```python
from build123d import *

# Parameters (mm, degrees)
BOSS_EXTRUDE1_DEPTH    = 24
F_6_0MM_DOWEL_HOLE1_D  = 6
SKETCH4_W              = 32.5
SKETCH4_H              = 30.5
CUT_EXTRUDE1_DEPTH     = 2
FILLET1_R              = 2
CUT_EXTRUDE2_DEPTH     = 57.482298112
FILLET2_R              = 4
SKETCH6_W              = 22.5
SKETCH6_H              = 20.5
CUT_EXTRUDE5_DEPTH     = 39.861935104
FILLET3_R              = 4
CUT_EXTRUDE6_DEPTH     = 39.861935104
FILLET4_R              = 4
M1_6_CLEARANCE_HOLE1_D = 1.8
CHAMFER1_SIZE          = 1


with BuildPart() as part:
    # Sketch1 → Boss-Extrude1 (new, symmetric)
    with BuildSketch(Plane(origin=(0, 0, 0), x_dir=(1, 0, 0), z_dir=(0, 1, 0))):
        with BuildLine():
            Line((25.5, 4), (-25.5, 4))
            ThreePointArc((-25.5, 4), (-29.5, 0), (-25.5, -4))
            Line((-25.5, -4), (25.5, -4))
            ThreePointArc((25.5, -4), (29.5, 0), (25.5, 4))
        make_face()
    extrude(amount=BOSS_EXTRUDE1_DEPTH, both=True)

    # Ø6.0mm Dowel Hole1 (through all)
    with Locations(Plane(origin=(0, -24, 0), x_dir=(-1, 0, 0), z_dir=(0, -1, 0))):
        with Locations((25.5, 0), (-25.5, 0)):
            Hole(F_6_0MM_DOWEL_HOLE1_D / 2)

    # Sketch4 → Cut-Extrude1 (cut)
    with BuildSketch(Plane(origin=(0, 0, 4), x_dir=(-1, 0, 0), z_dir=(0, 0, -1))):
        Rectangle(SKETCH4_W, SKETCH4_H)
    extrude(amount=CUT_EXTRUDE1_DEPTH, mode=Mode.SUBTRACT)

    # Fillet1
    fillet1_edges = [part.edges().sort_by_distance(p)[0] for p in [
        (-16.25, 15.25, 3),
        (16.25, 15.25, 3),
        (16.25, -15.25, 3),
        (-16.25, -15.25, 3),
    ]]
    fillet(fillet1_edges, radius=FILLET1_R)

    # Sketch5 → Cut-Extrude2 (cut, through all)
    with BuildSketch(Plane.XZ.offset(24)):
        with BuildLine():
            Line((21.5, 0), (-21.5, 0))
            ThreePointArc((-21.5, 0), (-22.671572875, -2.828427125), (-25.5, -4))
            Line((-25.5, -4), (25.5, -4))
            ThreePointArc((25.5, -4), (22.671572875, -2.828427125), (21.5, 0))
        make_face()
    extrude(amount=-CUT_EXTRUDE2_DEPTH, mode=Mode.SUBTRACT)

    # Fillet2
    fillet2_edges = [part.edges().sort_by_distance(p)[0] for p in [
        (21.5, 0, 0),
        (-21.5, 0, 0),
    ]]
    fillet(fillet2_edges, radius=FILLET2_R)

    # Sketch6 → Cut-Extrude5 (cut, through all)
    with BuildSketch(Plane.XY.offset(4)):
        Rectangle(SKETCH6_W, SKETCH6_H)
    extrude(amount=-CUT_EXTRUDE5_DEPTH, mode=Mode.SUBTRACT)

    # Fillet3
    fillet3_edges = [part.edges().sort_by_distance(p)[0] for p in [
        (11.25, -10.25, 1),
        (-11.25, -10.25, 1),
        (-11.25, 10.25, 1),
        (11.25, 10.25, 1),
    ]]
    fillet(fillet3_edges, radius=FILLET3_R)

    # Sketch7 → Cut-Extrude6 (cut, through all)
    with BuildSketch(Plane.XY.offset(4)):
        Polygon((18.57179677, 24), (-18.57179677, 24), (-13.82179677, 19.25), (13.82179677, 19.25), align=None)
        Polygon((-18.57179677, -24), (18.57179677, -24), (13.82179677, -19.25), (-13.82179677, -19.25), align=None)
    extrude(amount=-CUT_EXTRUDE6_DEPTH, mode=Mode.SUBTRACT)

    # Fillet4
    fillet4_edges = [part.edges().sort_by_distance(p)[0] for p in [
        (18.57179677, 24, 2),
        (13.82179677, 19.25, 2),
        (-13.82179677, 19.25, 2),
        (-18.57179677, 24, 2),
        (-18.57179677, -24, 2),
        (-13.82179677, -19.25, 2),
        (13.82179677, -19.25, 2),
        (18.57179677, -24, 2),
    ]]
    fillet(fillet4_edges, radius=FILLET4_R)

    # M1.6 Clearance Hole1 (through all)
    with Locations(Plane(origin=(0, 0, 0), x_dir=(-1, 0, 0), z_dir=(0, 0, -1))):
        with Locations((12.75, 12.75), (-12.75, 12.75), (-12.75, -12.75), (12.75, -12.75)):
            Hole(M1_6_CLEARANCE_HOLE1_D / 2)

    # Chamfer1
    chamfer1_edges = [part.edges().sort_by_distance(p)[0] for p in [
        (16.25, 0, 4),
        (0, -15.25, 4),
        (-16.25, 0, 4),
        (0, 15.25, 4),
        (15.664213562, -14.664213562, 4),
        (-15.664213562, 14.664213562, 4),
        (15.664213562, 14.664213562, 4),
        (-15.664213562, -14.664213562, 4),
    ]]
    chamfer(chamfer1_edges, length=CHAMFER1_SIZE)


solid = part.part
```
The model under review builds one solid part; all positions refer to its coordinate system, in mm. A direction names the side the tool comes from. Round coordinates to 2 decimals unless told otherwise and drop trailing zeros. Order: outer loops, then holes, each group sorted by start corner. A loop starts at its lowest first (then second) coordinate and runs counter-clockwise, first axis right, second up. Notation, with made-up numbers: (69, 63.25) - (91, 63.25) arc R27 cw to (91, 88.25) - close; hole circle Ø10 at (56, 8.5). An arc over 180 degrees is marked (long way). Answer in a Markdown table with one row per item.
(1) Clearance check with flat-ended pins moving along their axes: P1, Ø0.6, axis at x = 1.5, z = 1, coming from the -Y side; P2, Ø1.6, axis at x = -2, z = 1, coming from the +Y side; P3, Ø2, axis at x = -10, y = -17.5, coming from the -Z side. State where each tip first meets the part, or that it passes through.
Result set:
| item | result |
|---|---|
| P1 | stops at y = -19.25 |
| P2 | stops at y = 19.25 |
| P3 | stops at z = 0 |
(2) Take a section at B-B on y = -4.5. Write out the cut boundary in (x, z).
Result set:
| item | result |
|---|---|
| outline | (-25.5, 4) arc R4 ccw (long way) to (-22.04, -2) arc R4 cw to (-18.57, 0) - (-11.25, 0) - (-11.25, 2) - (-16.25, 2) - (-16.25, 3) - (-17.25, 4) - close; (11.25, 0) - (18.57, 0) arc R4 cw to (22.04, -2) arc R4 ccw (long way) to (25.5, 4) - (17.25, 4) - (16.25, 3) - (16.25, 2) - (11.25, 2) - close; hole circle Ø6 at (-25.5, 0); hole circle Ø6 at (25.5, 0) |
(3) For line 1 (X direction, y = -2.5, z = 0.25); line 2 (Y direction, x = -12.75, z = 1.25); line 3 (X direction, y = 13, z = -2.75), list the stretches that pass through material, from the lowest coordinate up. Write a range as from..to.
Result set:
| item | result |
|---|---|
| line 1 | x = -29.49..-28.49, -22.51..-11.25, 11.25..22.51, 28.49..29.49 |
| line 2 | y = -19.29..-13.65, -11.85..11.85, 13.65..19.29 |
| line 3 | x = -28.4..-26.7, -24.3..-22.6, 22.6..24.3, 26.7..28.4 |
(4) Take a section at A-A on x = 5. Write out the cut boundary in (y, z), plus the area to 3 significant figures.
Result set:
| item | result |
|---|---|
| outline | (-19.25, 0) - (-10.25, 0) - (-10.25, 2) - (-15.25, 2) - (-15.25, 3) - (-16.25, 4) - (-19.25, 4) - close; (10.25, 0) - (19.25, 0) - (19.25, 4) - (16.25, 4) - (15.25, 3) - (15.25, 2) - (10.25, 2) - close |
| area | 51.0 mm2 |
(5) Take a section at C-C on z = 1.25. Count the separate pieces of the cut face and the enclosed holes in it, plus the area to 3 significant figures.
Result set:
| item | result |
|---|---|
| separate pieces | 3 |
| enclosed holes | 5 |
| area | 1,520 mm2 |
(6) Machinability: for faces 4 (the face through (-18.68, 23.69, 1.79)), 5 (the face through (10.109, 9.047, 0.986)), 6 (the face through (-15.953, -14.916, 3.382)), 7 (the face through (13.716, -19.563, 1.972)), which of the approach directions +Z, -Z, +X, -X, +Y, -Y give a long, thin tool a straight path to every point of the face, cutting with its end or side? Answer none if there is none.
Result set:
| item | result |
|---|---|
| face 4 | +Z, -Z, +Y |
| face 5 | +Z, -Z |
| face 6 | +Z |
| face 7 | +Z, -Z, -Y |
(7) Mouldability with a two-part tool opening along X and no side actions: class faces 1 (the face through (13.68, 19.55, 1.97)), 2 (the face through (15.953, 14.916, 3.382)), 3 (the face through (23, -24, 2)) as released by +X, released by -X, zero draft, split by the parting line, or undercut.
Result set:
| item | result |
|---|---|
| face 1 | undercut |
| face 2 | undercut |
| face 3 | zero draft |
